Model file for the job. Use its own axes, mm. A direction names the side the tool comes from. Coordinates: 2 decimals unless noted, no trailing zeros. Order: outer loops, then holes, each group sorted by start corner. A loop starts at its lowest first (then second) coordinate and runs counter-clockwise, first axis right, second up. Notation, with made-up numbers: (34, -27.75) -> (39, -27.75) arc R15 cw to (39, -18.75) -> close; hole circle Ø7 at (62.5, 52). An arc over 180 degrees is marked (long way). Write item = value, one per line. Start each with the question number.
Q1. 3-axis set-ups, long thin cutter, end or side, ignore diameter. For faces 1 (the face through (1.836, 0.531, 4.765)), 2 (the face through (0, 5, -4)): which of +Z, -Z, +X, -X, +Y, -Y reach the whole face in a straight line?
Q2. Cut at A-A, the plane y = 131. List the corners of the cut face in (x, z), plus the area to 3 significant figures.
Q3. Cut at B-B, the plane y = 89. List the corners of the cut face in (x, z) (3 decimals).
Q4. Wall check: line 1 (Z direction, x = 0.75, y = 70); line 2 (Z direction, x = 4.75, y = 68); line 3 (X direction, y = 25, z = 2.5). Give the ranges that are in metal, low to high. Write a range as from..to.
Q5. Mould opens along Z. For faces 3 (the face through (0, 5, 4)), 4 (the face through (-4.1, 5, 0)), 5 (the face through (4.9, 12, 0)), 6 (the face through (-0.9, 136.42, -2.86)) say: +Z half, -Z half, draft (parallel to the pull), parting line (faces both ways), or undercut.
Q6. Flat gauge pins, fed straight in: pin 1 (2 mm diameter, centred on y = 8, z = 1.5, fed in from +X); pin 2 (2 mm diameter, centred on x = 3, y = 78, fed in from +Z); pin 3 (5 mm diameter, centred on y = 61.5, z = -3.5, fed in from +X). Where does each tip first touch, or does it go through?
from build123d import *

# Parameters (mm, degrees)
FILLET1_R               = 2
FILLET2_R               = 100
CUT_EXTRUDE1_DEPTH      = 156.272341396
CUT_EXTRUDE1_DEPTH_BACK = 156.272341396
SKETCH3_W               = 11
SKETCH3_H               = 8
CUT_EXTRUDE2_DEPTH      = 10.6
FILLET3_R               = 0.5


with BuildPart() as part:
    # Sketch1 → Revolve1 (revolve)
    with BuildSketch(Plane.XY, mode=Mode.PRIVATE) as revolve1_sk:
        Polygon((6.5, 0), (6.5, 75), (3, 115), (3, 155), (0, 155), (0, 0), align=None)
    revolve(revolve1_sk.sketch.rotate(Axis((0, 0, 0), (0, 1, 0)), 90), axis=Axis((0, 0, 0), (0, 1, 0)))

    # Fillet1
    fillet1_edges = [part.edges().sort_by_distance(p)[0] for p in [
        (0, 155, 3),
    ]]
    fillet(fillet1_edges, radius=FILLET1_R)

    # Fillet2
    # the kernel refuses this fillet: 100 mm, written as the material it adds along each edge
    with BuildSketch(Plane(origin=(0, 115, 0), x_dir=(0, 0, -1), z_dir=(1, 0, 0))) as fillet2_piece_1:
        with BuildLine():
            CenterArc((3 + FILLET2_R, FILLET2_R * 0.0436665788079), FILLET2_R, 180, 5.000644598)
            Line((3 + FILLET2_R * 0.00380628250389, -FILLET2_R * 0.043500371473), (3 - FILLET2_R * 0.016117591846, -FILLET2_R * 0.0452437104786))
            Line((3 - FILLET2_R * 0.016117591846, -FILLET2_R * 0.0452437104786), (3 - FILLET2_R * 0.0199238743499, -FILLET2_R * 0.00174333900562))
            Line((3 - FILLET2_R * 0.0199238743499, -FILLET2_R * 0.00174333900562), (3 - FILLET2_R * 0.02, 0))
            Line((3 - FILLET2_R * 0.02, 0), (3 - FILLET2_R * 0.02, FILLET2_R * 0.0436665788079))
            Line((3 - FILLET2_R * 0.02, FILLET2_R * 0.0436665788079), (3, FILLET2_R * 0.0436665788079))
        make_face()
    revolve(axis=Axis((0, 115, 0), (0, 1, 0)))
    # the kernel refuses this fillet: 100 mm, written as the material it takes off along each edge
    with BuildSketch(Plane(origin=(0, 75, 0), x_dir=(0, 0, -1), z_dir=(1, 0, 0))) as fillet2_2_piece_1:
        with BuildLine():
            CenterArc((6.5 - FILLET2_R, -FILLET2_R * 0.0436665788079), FILLET2_R, 0, 5.000644598)
            Line((6.5, -FILLET2_R * 0.0436665788079), (6.5 + FILLET2_R * 0.02, -FILLET2_R * 0.0436665788079))
            Line((6.5 + FILLET2_R * 0.02, -FILLET2_R * 0.0436665788079), (6.5 + FILLET2_R * 0.02, FILLET2_R * 0.000873331576158))
            Line((6.5 + FILLET2_R * 0.02, FILLET2_R * 0.000873331576158), (6.5 + FILLET2_R * 0.016117591846, FILLET2_R * 0.0452437104786))
            Line((6.5 + FILLET2_R * 0.016117591846, FILLET2_R * 0.0452437104786), (6.5 - FILLET2_R * 0.00380628250389, FILLET2_R * 0.043500371473))
        make_face()
    revolve(axis=Axis((0, 75, 0), (0, 1, 0)), mode=Mode.SUBTRACT)

    # Sketch2 → Cut-Extrude1 (cut, two sides: drawn at the far end of the back side and taken through both)
    with BuildSketch(Plane.XY.offset(-CUT_EXTRUDE1_DEPTH_BACK)):
        with BuildLine():
            Line((6.5, 14), (4.9, 12.4))
            Line((4.9, 12.4), (4.9, 5.4))
            ThreePointArc((4.9, 5.4), (3.318376618, 1.581623382), (-0.5, 0))
            Line((-0.5, 0), (6.5, 0))
            Line((6.5, 0), (6.5, 14))
        make_face()
    extrude(amount=CUT_EXTRUDE1_DEPTH + CUT_EXTRUDE1_DEPTH_BACK, mode=Mode.SUBTRACT)

    # Sketch3 → Cut-Extrude2 (cut)
    with BuildSketch(Plane(origin=(0, 0, 0), x_dir=(1, 0, 0), z_dir=(0, 1, 0))):
        with Locations((1.4, 0)):
            Rectangle(SKETCH3_W, SKETCH3_H)
    extrude(amount=CUT_EXTRUDE2_DEPTH, mode=Mode.SUBTRACT)

    # Fillet3
    fillet3_edges = [part.edges().sort_by_distance(p)[0] for p in [
        (-6.5, 0, 0),
        (3.349776633, 1.613283763, 5.570367722),
        (3.507900773, 1.781059372, -5.47216888),
        (4.9, 8.9, -4.270831301),
        (4.9, 8.9, 4.270831301),
    ]]
    fillet(fillet3_edges, radius=FILLET3_R)


solid = part.part
Here are the results:
q1.face_1 = +Z, -Z, +X, -Y
q1.face_2 = +X, -Y
q2.outline = circle Ø6 at (0, 0)
q2.area = 28.3 mm²
q3.outline = circle Ø10.55 at (0, 0)
q4.line_1 = -6.46..6.46
q4.line_2 = -4.44..4.44
q4.line_3 = -6..6
q5.face_3 = undercut
q5.face_4 = undercut
q5.face_5 = draft
q5.face_6 = parting line
q6.pin_1 = -4.1
q6.pin_2 = 5.91
q6.pin_3 = 6.42
